Input: part model. Units: mm. Frame: model coordinates. Give positions to 0.01 mm unless a question says otherwise; leave off trailing zeros. Loops run counter-clockwise (first coordinate to the right, second up) from the corner with the lowest first, then second, coordinate; pieces in that order, holes last. Notation, with made-up numbers: (32.25, 89) - (59.25, 89) arc R20 ccw to (59.25, 112) - close; hole circle Ø5 at (12.5, -10). An arc over 180 degrees is marked (long way). Answer as a JSON object with one key per item and string values. Group by question number.
(1) Material intervals for L1, parallel to Y at x = -32.5, z = 0.3; L2, parallel to X at y = 10.25, z = 0.35; L3, parallel to Y at x = 17.5, z = 1.05, sorted ascending.
(2) Section query A-A (x = -9). Return loops of the section in (y, z).
(3) Section query B-B (x = 2.5). Return loops of the section in (y, z), plus the area to 3 significant figures.
(4) Pin query (flat end, axial travel): P1, Ø1.5, axis at x = 32.5, y = -10.25, coming from the +Z side; P2, Ø2, axis at y = 8.5, z = -2, coming from the +X side; P3, Ø1, axis at y = 6.5, z = -1, coming from the +X side; P4, Ø1.5, axis at x = 15.5, z = -2, coming from the -Y side. Return the tip coordinate at first contact, or that it passes through.
Autodesk Inventor part; units mm, degrees
ref_plane "YZ Plane" through (0, 0, 0) normal (1, 0, 0) x (0, 1, 0)
ref_plane "XZ Plane" through (0, 0, 0) normal (0, 1, 0) x (-1, 0, 0)
ref_plane "XY Plane" through (0, 0, 0) normal (0, 0, 1) x (1, 0, 0)
sketch "Sketch1" plane through (0, 0, 0) normal (0, 0, 1) x (1, 0, 0)
  line L0 (-35.5, 13.25) -> (35.5, 13.25)
  line L1 (35.5, 13.25) -> (35.5, -13.25)
  line L2 (35.5, -13.25) -> (-35.5, -13.25)
  line L3 (-35.5, -13.25) -> (-35.5, 13.25)
  point P0 (0, 0)
  dimension "d0" = 26.5
  dimension "d1" = 71
  dimension "d2" = 35.5
  dimension "d3" = 13.25
extrude "Extrusion1" add sketch "Sketch1" along normal blind 1.2
fillet "Fillet1" radius 3.25 4 edges at (-35.5, 13.25, 0.6) (-35.5, -13.25, 0.6) (35.5, -13.25, 0.6) (35.5, 13.25, 0.6)
sketch "Sketch2" plane through (0, 0, 1.2) normal (0, 0, 1) x (1, 0, 0)
  line L0 (32.25, 13.25) -> (-32.25, 13.25)
  line L1 (-35.5, 10) -> (-35.5, -10)
  line L2 (-32.25, -13.25) -> (32.25, -13.25)
  line L3 (35.5, -10) -> (35.5, 10)
  point P0 (0, 0)
  point P1 (-32.5, 10.25)
  point P2 (32.5, 10.25)
  point P3 (32.5, -10.25)
  point P4 (-32.5, -10.25)
  dimension "d7" = 3
  dimension "d8" = 3
  dimension "d9" = 3
  dimension "d10" = 3
  dimension "d11" = 3
  dimension "d12" = 3
  dimension "d13" = 3
  dimension "d14" = 3
hole "Hole1" at (-32.5, 10.25, 1.2) at (32.5, 10.25, 1.2) at (32.5, -10.25, 1.2) at (-32.5, -10.25, 1.2) direction (0, 0, -1) diameter 2.5 depth 4 tip angle 118 countersink diameter 4 countersink angle 90
sketch "Sketch4" plane through (0, 0, 1.2) normal (0, 0, 1) x (1, 0, 0)
  line L0 (-11, -3.25) -> (-1, -3.25)
  line L1 (-1, -3.25) -> (-1, -7.25)
  line L2 (-1, -7.25) -> (-11, -7.25)
  line L3 (-11, -7.25) -> (-11, -3.25)
  line L4 (-35.5, 10) -> (-35.5, -10)
  line L5 (-32.25, -13.25) -> (32.25, -13.25)
  point P0 (0, 0)
  dimension "d28" = 24.5
  dimension "d29" = 34.5
  dimension "d30" = 6
  dimension "d31" = 10
extrude "Extrusion3" cut sketch "Sketch4" against normal blind 2
sketch "Sketch5" plane through (0, 0, 1.2) normal (0, 0, 1) x (1, 0, 0)
  line L0 (6.5, 1.75) -> (24.5, 1.75)
  line L1 (24.5, 1.75) -> (24.5, -5.25)
  line L2 (24.5, -5.25) -> (6.5, -5.25)
  line L3 (6.5, -5.25) -> (6.5, 1.75)
  line L4 (35.5, -10) -> (35.5, 10)
  line L5 (-32.25, -13.25) -> (32.25, -13.25)
  point P0 (0, 0)
  dimension "d34" = 11
  dimension "d35" = 29
  dimension "d36" = 15
  dimension "d37" = 8
extrude "Extrusion4" cut sketch "Sketch5" against normal blind 2
chamfer "Chamfer1" distance 2 angle 45 2 edges at (6.5, -5.25, 0.6) (24.5, -5.25, 0.6)
fillet "Fillet2" radius 1 4 edges at (-11, -3.25, 0.6) (-11, -7.25, 0.6) (-1, -7.25, 0.6) (-1, -3.25, 0.6)
sketch "Sketch7" plane through (0, 0, 1.2) normal (0, 0, 1) x (1, 0, 0)
  line L0 (0, 3.85) -> (28.6, 3.85)
  line L1 (28.6, 3.85) -> (28.6, -9.35)
  line L2 (28.6, -9.35) -> (0, -9.35)
  line L3 (0, -9.35) -> (0, 3.85)
  line L4 (-32.25, -13.25) -> (32.25, -13.25)
  line L5 (35.5, -10) -> (35.5, 10)
  point P0 (0, 0)
  dimension "d56" = 3.9
  dimension "d57" = 6.9
  dimension "d58" = 17.1
  dimension "d59" = 35.5
extrude "Extrusion6" cut sketch "Sketch7" against normal blind 2
fillet "Fillet3" radius 6 4 edges at (0, 3.85, 0.6) (0, -9.35, 0.6) (28.6, 3.85, 0.6) (28.6, -9.35, 0.6)
sketch "Sketch8" plane through (0, 0, 1.2) normal (0, 0, 1) x (1, 0, 0)
  line L0 (-26.5, -3.25) -> (-16.5, -3.25)
  line L1 (-16.5, -3.25) -> (-16.5, -7.25)
  line L2 (-16.5, -7.25) -> (-26.5, -7.25)
  line L3 (-26.5, -7.25) -> (-26.5, -3.25)
  line L4 (-35.5, 10) -> (-35.5, -10)
  line L5 (-10, -3.25) -> (-2, -3.25)
  line L6 (-2, -7.25) -> (-10, -7.25)
  point P0 (0, 0)
  dimension "d63" = 9
  dimension "d64" = 19
extrude "Extrusion7" cut sketch "Sketch8" against normal blind 2
fillet "Fillet4" radius 1 4 edges at (-26.5, -3.25, 0.6) (-26.5, -7.25, 0.6) (-16.5, -7.25, 0.6) (-16.5, -3.25, 0.6)
sketch "Sketch9" plane through (0, 0, 1.2) normal (0, 0, 1) x (1, 0, 0)
  line L0 (-1, -4.25) -> (-1, -6.25)
  line L1 (-11, -6.25) -> (-11, -4.25)
  line L2 (-26.5, -6.25) -> (-26.5, -4.25)
  line L3 (-16.5, -4.25) -> (-16.5, -6.25)
  line L4 (-35.5, 10) -> (-35.5, -10)
  point P0 (0, 0)
  dimension "d68" = 10
  dimension "d69" = 10
  dimension "d70" = 24.5
  dimension "d71" = 34.5
sketch "Sketch10" plane through (0, 0, 0) normal (0, 0, -1) x (-1, 0, 0)
  line L0 (-29.5, 8.25) -> (29.5, 8.25)
  line L1 (29.5, 8.25) -> (29.5, 6.7885)
  line L2 (29.5, 6.7885) -> (-29.5, 6.7885)
  line L3 (-29.5, 6.7885) -> (-29.5, 8.25)
  line L4 (-35.5, -10) -> (-35.5, 10)
  line L5 (35.5, 10) -> (35.5, -10)
  line L6 (-32.25, 13.25) -> (32.25, 13.25)
  point P0 (0, 0)
  dimension "d72" = 1.4615
  dimension "d73" = 6
  dimension "d74" = 6
  dimension "d75" = 5
extrude "Extrusion8" add sketch "Sketch10" along normal blind 3
fillet "Fillet5" radius 1 2 edges at (0, 6.7885, 0) (0, 8.25, 0)
chamfer "Chamfer4" distance 3 angle 45 2 edges at (29.5, 7.5192, -3) (-29.5, 7.5192, -3)
properties part number "cover-slave"
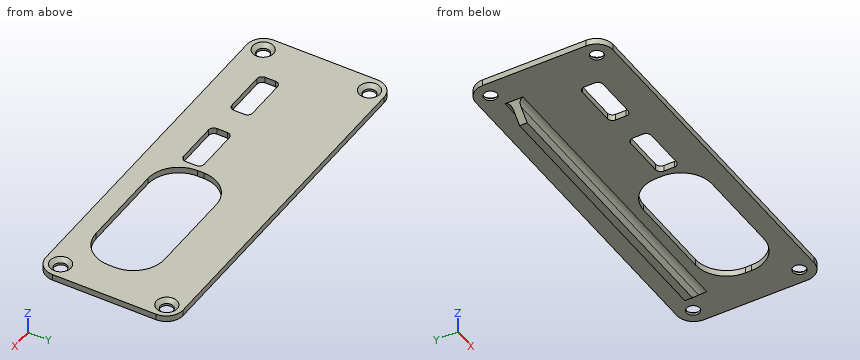
Recorded:
{
 "1": {"L1": "y = -13.24 to -11.5, -9 to 9, 11.5 to 13.24", "L2": "x = -35.49 to -33.75, -31.25 to 31.25, 33.75 to 35.49", "L3": "y = -13.25 to -9.35, 3.85 to 13.25"},
 "2": {"outline": "(-13.25, 0) - (-7.25, 0) - (-7.25, 1.2) - (-13.25, 1.2) - close; (-3.25, 0) - (5.79, 0) arc R1 cw to (6.79, -1) - (6.79, -3) - (8.25, -3) - (8.25, -1) arc R1 cw to (9.25, 0) - (13.25, 0) - (13.25, 1.2) - (-3.25, 1.2) - close"},
 "3": {"outline": "(-13.25, 0) - (-8.22, 0) - (-8.22, 1.2) - (-13.25, 1.2) - close; (2.72, 0) - (5.79, 0) arc R1 cw to (6.79, -1) - (6.79, -3) - (8.25, -3) - (8.25, -1) arc R1 cw to (9.25, 0) - (13.25, 0) - (13.25, 1.2) - (2.72, 1.2) - close", "area": "23.5 mm^2"},
 "4": {"P1": "passes through", "P2": "stops at x = 28.47", "P3": "stops at x = 28.97", "P4": "stops at y = 6.79"}
}
